Source: CAD feature listing. Evaluate the final solid. Frame: model axes, mm. Face numbers are marked on the shaded views. A direction names the side the tool comes from. Round coordinates to 2 decimals unless told otherwise and drop trailing zeros. Loops run counter-clockwise (first coordinate to the right, second up) from the corner with the lowest first, then second, coordinate; pieces in that order, holes last. Notation, with made-up numbers: M 81,46.25 L 87,46.25 A14 cw 87,53.25 Z; hole C 70,27.5 d2. An arc over 180 degrees is marked long. Answer as CSV lines item,"result". Start each with the question number.
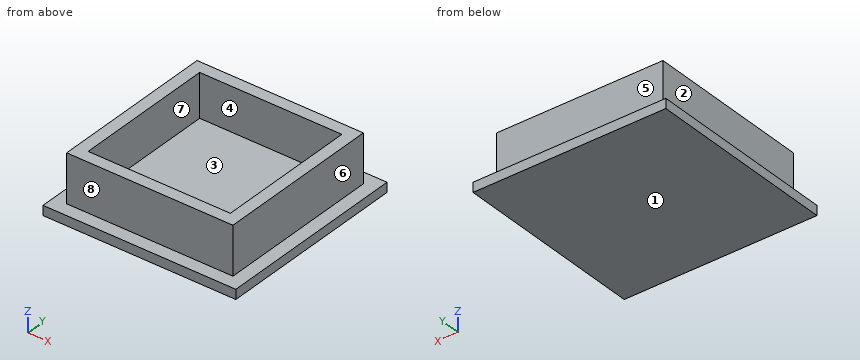
```python
from build123d import *

# Parameters (mm, degrees)
SKETCH_W     = 40
SKETCH_H     = 40
PAD_DEPTH    = 2
SKETCH001_W  = 34.5
SKETCH001_H  = 34.5
PAD001_DEPTH = 10
SKETCH002_W  = 29.5
SKETCH002_H  = 29.5
POCKET_DEPTH = 9


with BuildPart() as part:
    # Sketch → Pad (new body)
    with BuildSketch(Plane.XY):
        Rectangle(SKETCH_W, SKETCH_H)
    extrude(amount=PAD_DEPTH)

    # Sketch001 (on Face6 of Pad) → Pad001 (join)
    with BuildSketch(Plane.XY.offset(2)):
        Rectangle(SKETCH001_W, SKETCH001_H)
    extrude(amount=PAD001_DEPTH)

    # Sketch002 (on Face11 of Pad001) → Pocket (cut)
    with BuildSketch(Plane.XY.offset(12)):
        Rectangle(SKETCH002_W, SKETCH002_H)
    extrude(amount=-POCKET_DEPTH, mode=Mode.SUBTRACT)


solid = part.part
```
1) Mould query, pull axis X, two halves, no side actions, for the marked faces 1, 2, 3 and 4. Classes: pulls with the +X half, pulls with the -X half, needs draft (parallel to the pull), parting line crosses it, or undercut.
2) Section A-A, the plane x = -9.5. Return loops of the section in (y, z).
3) Contact query for flat-ended pins moving along their axis: pin 1 Ø4.5 at (y, z) = (5, 6) entering from +X; pin 2 Ø5 at (x, z) = (6, 5.5) entering from -Y; pin 3 Ø2.5 at (x, z) = (5, 6) entering from +Y. Output: stop coordinate, or through.
4) Access query for the marked faces 5, 6, 7 and 8. Directions: +Z, -Z, +X, -X, +Y, -Y. A direction counts if a zero-diameter tool reaches every point of the face in a straight line with its end or side. Return the directions, or none.
5) Section B-B, the plane z = 10.75. Return loops of the section in (x, y), and give its area (3 significant figures).
6) Ray query, line 1 along X through (y, z) = (-5, 3.5); line 2 along Y through (x, z) = (16.5, 7). Return the intervals inside material, ascending.
Findings below:
1,face 1,"needs draft"
1,face 2,"pulls with the -X half"
1,face 3,"undercut"
1,face 4,"undercut"
2,outline,"M -20,0 L 20,0 L 20,2 L 17.25,2 L 17.25,12 L 14.75,12 L 14.75,3 L -14.75,3 L -14.75,12 L -17.25,12 L -17.25,2 L -20,2 Z"
3,pin 1,"x = 17.25"
3,pin 2,"y = -17.25"
3,pin 3,"y = 17.25"
4,face 5,"+Z, +X, -X, +Y"
4,face 6,"+Z, +X, +Y, -Y"
4,face 7,"+Z"
4,face 8,"+Z, +X, -X, -Y"
5,outline,"M -17.25,-17.25 L 17.25,-17.25 L 17.25,17.25 L -17.25,17.25 Z; hole M -14.75,-14.75 L 14.75,-14.75 L 14.75,14.75 L -14.75,14.75 Z"
5,area,"320 mm²"
6,line 1,"-17.25 to -14.75, 14.75 to 17.25"
6,line 2,"-17.25 to 17.25"
